The listing builds one solid part. Answer for the finished solid, in the listing's coordinates (mm). A direction names the side the tool comes from. Coordinates: 2 decimals unless noted, no trailing zeros. Loops run counter-clockwise (first coordinate to the right, second up) from the corner with the lowest first, then second, coordinate; pieces in that order, holes last. Notation, with made-up numbers: (28.5, 43) - (51.5, 43) arc R36 ccw to (51.5, 81) - close; hole circle Ø4 at (-1.5, 7.25). An arc over 180 degrees is marked (long way). Put each result on its own line as item: value.
```python
from build123d import *

# Parameters (mm, degrees)
F0_W     = 15
F0_H     = 15
F1_DEPTH = 20
F3_DEPTH = 5
F5_DEPTH = 5
F7_DEPTH = 5
F9_DEPTH = 5


with BuildPart() as f1:
    # F0 (on Top) → F1 (new body)
    with BuildSketch(Plane.XY):
        Rectangle(F0_W, F0_H)
    extrude(amount=F1_DEPTH)

    # F2 (on face) → F3 (cut)
    with BuildSketch(Plane.XY.offset(20)):
        Polygon((3.3, -1.905256), (3.3, 1.905256), (0, 3.810512), (-3.3, 1.905256), (-3.3, -1.905256), (0, -3.810512), align=None)
    extrude(amount=-F3_DEPTH, mode=Mode.SUBTRACT)

    # F4 (on face) → F5 (cut)
    with BuildSketch(Plane.XY.offset(15)):
        Polygon((3.2, -1.847521), (3.2, 1.847521), (0, 3.695042), (-3.2, 1.847521), (-3.2, -1.847521), (0, -3.695042), align=None)
    extrude(amount=-F5_DEPTH, mode=Mode.SUBTRACT)

    # F6 (on face) → F7 (cut)
    with BuildSketch(Plane.XY.offset(10)):
        Polygon((3.1, -1.789786), (3.1, 1.789786), (0, 3.579572), (-3.1, 1.789786), (-3.1, -1.789786), (0, -3.579572), align=None)
    extrude(amount=-F7_DEPTH, mode=Mode.SUBTRACT)

    # F8 (on face) → F9 (cut)
    with BuildSketch(Plane.XY.offset(5)):
        Polygon((3, -1.732051), (3, 1.732051), (0, 3.464102), (-3, 1.732051), (-3, -1.732051), (0, -3.464102), align=None)
    extrude(amount=-F9_DEPTH, mode=Mode.SUBTRACT)


solid = f1.part
```
1) The part is cut by section D-D (z = 6.5). Give the vertices of the cut face in (x, y), and give its area (3 significant figures).
Found:
outline: (-7.5, -7.5) - (7.5, -7.5) - (7.5, 7.5) - (-7.5, 7.5) - close; hole (-3.1, -1.79) - (0, -3.58) - (3.1, -1.79) - (3.1, 1.79) - (0, 3.58) - (-3.1, 1.79) - close
area: 192 mm^2
2) The part is cut by section C-C (x = 1.75). Give the vertices of the cut face in (y, z), and give its area (3 significant figures).
Found:
outline: (-7.5, 0) - (-2.45, 0) - (-2.45, 5) - (-2.57, 5) - (-2.57, 10) - (-2.68, 10) - (-2.68, 15) - (-2.8, 15) - (-2.8, 20) - (-7.5, 20) - close; (2.45, 0) - (7.5, 0) - (7.5, 20) - (2.8, 20) - (2.8, 15) - (2.68, 15) - (2.68, 10) - (2.57, 10) - (2.57, 5) - (2.45, 5) - close
area: 195 mm^2
3) Straight lines are drawn through the part: L1, parallel to X at y = 1, z = 4.25; L2, parallel to Z at x = -3.25, y = 0.25; L3, parallel to Y at x = 0.25, z = 6.5. For each, find the intervals that lie inside material, in ascending order. Write a range as [from, to].
Found:
L1: x = [-7.5, -3], [3, 7.5]
L2: z = [0, 15]
L3: y = [-7.5, -3.44], [3.44, 7.5]
4) The part is cut by section B-B (z = 13.75). Give the vertices of the cut face in (x, y).
Found:
outline: (-7.5, -7.5) - (7.5, -7.5) - (7.5, 7.5) - (-7.5, 7.5) - close; hole (-3.2, -1.85) - (0, -3.7) - (3.2, -1.85) - (3.2, 1.85) - (0, 3.7) - (-3.2, 1.85) - close
5) For faces 1 (the face through (-1.5, 2.6, 2.5)), 2 (the face through (-3.3, 0, 18)), determine the directions among +Z, -Z, +X, -X, +Y, -Y from which every point of the face is accessible in a straight line to the end or side of a thin tool.
Found:
face 1: +Z, -Z
face 2: +Z
6) This flat-tipped pin is pushed along its axis until it touches: pin 1 (2 mm diameter, centred on x = -1, y = 0, fed in from +Z). Where does it stop, or does it pass through?
Found:
pin 1: passes through
7) The part is cut by section A-A (y = -0.5). Give the vertices of the cut face in (x, z).
Found:
outline: (-7.5, 0) - (-3, 0) - (-3, 5) - (-3.1, 5) - (-3.1, 10) - (-3.2, 10) - (-3.2, 15) - (-3.3, 15) - (-3.3, 20) - (-7.5, 20) - close; (3, 0) - (7.5, 0) - (7.5, 20) - (3.3, 20) - (3.3, 15) - (3.2, 15) - (3.2, 10) - (3.1, 10) - (3.1, 5) - (3, 5) - close
8) For a pull along X with two mould halves and no side action, classify faces 3 (the face through (1.5, -2.6, 2.5)), 4 (the face through (-2, 3, 20)), 5 (the face through (-7.5, 0, 10)) as pulls with the +X half, pulls with the -X half, needs draft (parallel to the pull), parting line crosses it, or undercut.
Found:
face 3: undercut
face 4: needs draft
face 5: pulls with the -X half
